Read the model definition and answer for the solid it produces. Units are mm, in the model's axes. Face numbers are marked on the shaded views. A direction names the side the tool comes from. Coordinates: 2 decimals unless noted, no trailing zeros. Write each loop counter-clockwise with the first axis right and the second up, starting at its lowest first coordinate (ties: lowest second). Pieces come first, ordered by that corner, then holes. Notation, with made-up numbers: M -16,30.25 L 13,30.25 A17 ccw 13,45.25 Z; hole C 52,-12 d4. An arc over 180 degrees is marked long. Write item = value, one per line.
from build123d import *

# Parameters (mm, degrees)
BOSS_EXTRUDE1_DEPTH            = 50.8
SKETCH4_W                      = 1.5875
SKETCH4_H                      = 12.7
BOSS_EXTRUDE2_DEPTH            = 9.525
FILLET2_R                      = 3.175
F_3_16_0_1875_DIAMETER_HOLE1_D = 4.7625
CHAMFER1_SIZE                  = 6.35


with BuildPart() as part:
    # Sketch1 → Boss-Extrude1 (new body)
    with BuildSketch(Plane.XY):
        Polygon((17.4625, 9.525), (17.4625, 1.5875), (1.5875, 1.5875), (1.5875, 9.525), (0, 9.525), (0, 0), (19.05, 0), (19.05, 9.525), align=None)
    extrude(amount=BOSS_EXTRUDE1_DEPTH)

    # Sketch4 → Boss-Extrude2 (add)
    with BuildSketch(Plane(origin=(0, 9.525, 0), x_dir=(1, 0, 0), z_dir=(0, 1, 0))):
        with Locations((0.79375, -6.35)):
            Rectangle(SKETCH4_W, SKETCH4_H)
        with Locations((18.25625, -6.35)):
            Rectangle(SKETCH4_W, SKETCH4_H)
    extrude(amount=BOSS_EXTRUDE2_DEPTH)

    # Fillet2
    fillet2_edges = [part.edges().sort_by_distance(p)[0] for p in [
        (0.79375, 9.525, 12.7),
        (0.79375, 19.05, 12.7),
        (0.79375, 19.05, 0),
        (18.25625, 9.525, 12.7),
        (18.25625, 19.05, 12.7),
        (18.25625, 19.05, 0),
    ]]
    fillet(fillet2_edges, radius=FILLET2_R)

    # 3/16 (0.1875) Diameter Hole1 (through all)
    with Locations(Plane(origin=(19.05, 0, 0), x_dir=(0, 0, -1), z_dir=(1, 0, 0))):
        with Locations((-6.35, 14.2875), (4.115757827, 15.875)):
            Hole(F_3_16_0_1875_DIAMETER_HOLE1_D / 2)

    # Chamfer1
    # the kernel refuses this chamfer: 6.35 mm, written as the material it takes off along each edge
    with BuildSketch(Plane(origin=(-16.330186974, 0, 0), x_dir=(0, 0.9996219169112966, -0.02749587661058637), z_dir=(1, 0, 0))) as chamfer1_piece_1:
        Polygon((CHAMFER1_SIZE * 0.999621916911, CHAMFER1_SIZE * 0.0274958766106), (-CHAMFER1_SIZE * 0.0274958766106, CHAMFER1_SIZE * 0.999621916911), (0, 0), align=None)
    extrude(amount=51.710373947, mode=Mode.SUBTRACT)


solid = part.part
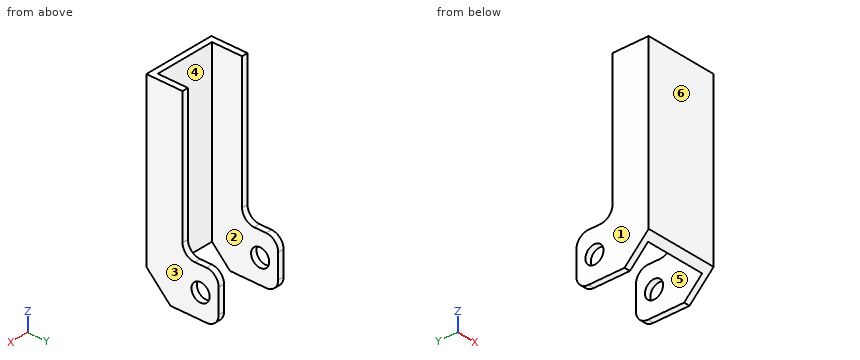
Item 1: For a pull along X with two mould halves and no side action, classify the marked faces 3, 4, 5 and 6 as released by +X, released by -X, zero draft, split by the parting line, or undercut.
Worked answers:
face_3 = released by +X
face_4 = undercut
face_5 = undercut
face_6 = zero draft
Item 2: Find section C-C (x = 8.5). Determine the outline of the cut face in (y, z).
Worked answers:
outline = M 0,6.35 L 1.59,4.76 L 1.59,50.8 L 0,50.8 Z
Item 3: Which of the six approach directions +Z, -Z, +X, -X, +Y, -Y give full straight-line access (tool end or side, diameter ignored) to the marked faces 1 and 2?
Worked answers:
face_1 = +Z, -Z, -X, +Y, -Y
face_2 = +Z, -Z, +Y
Item 4: Consider line 1 along Y through (x, z) = (0.95, 6.35); line 2 along X through (y, z) = (7, 37); line 3 along Y through (x, z) = (9.5, 39). Determine where each line is inside the solid, lowest interval first. Write a range as from..to.
Worked answers:
line_1 = 0..11.91, 16.67..19.05
line_2 = 0..1.59, 17.46..19.05
line_3 = 0..1.59
Item 5: Flat-ended cylindrical pins translate along their axes: pin 1 (1.7 mm diameter, centred on x = 1, z = 27, fed in from +Y) (3 decimals); pin 2 (0.5 mm diameter, centred on x = 18, y = 15, fed in from +Z); pin 3 (10 mm diameter, centred on x = 7.5, y = 8.5, fed in from +Z); pin 4 (1.5 mm diameter, centred on x = 5.5, z = 34.5, fed in from +Y). Find the tip coordinate at first contact, or state that the pin passes through.
Worked answers:
pin_1 = 9.525
pin_2 = 12.7
pin_3 = through
pin_4 = 1.59
Item 6: Find section B-B (y = 13.25). Determine the outline of the cut face in (x, z).
Worked answers:
outline = M 0,0 L 1.59,0 L 1.59,4.21 L 0,4.21 Z; M 0,8.49 L 1.59,8.49 L 1.59,12.7 L 0,12.7 Z; M 17.46,0 L 19.05,0 L 19.05,4.21 L 17.46,4.21 Z; M 17.46,8.49 L 19.05,8.49 L 19.05,12.7 L 17.46,12.7 Z
